The drawing under review shows one solid part. Ordinate dimensions are in mm from its lowest x, y, z. A direction names the side the tool comes from. Give positions to 0.01 mm unless a question says otherwise; leave off trailing zeros. Write each loop counter-clockwise with the first axis right and the second up, starting at its lowest first coordinate (ties: lowest second). Pieces come first, ordered by that corner, then holes. Notation, with made-up numbers: M 88,55.5 L 141,55.5 A18 ccw 141,77.5 Z; hole C -15.5,-28 d11. An arc over 180 degrees is marked long. Write each question's results on one line, items separated by ' | '. Start each with the question number.
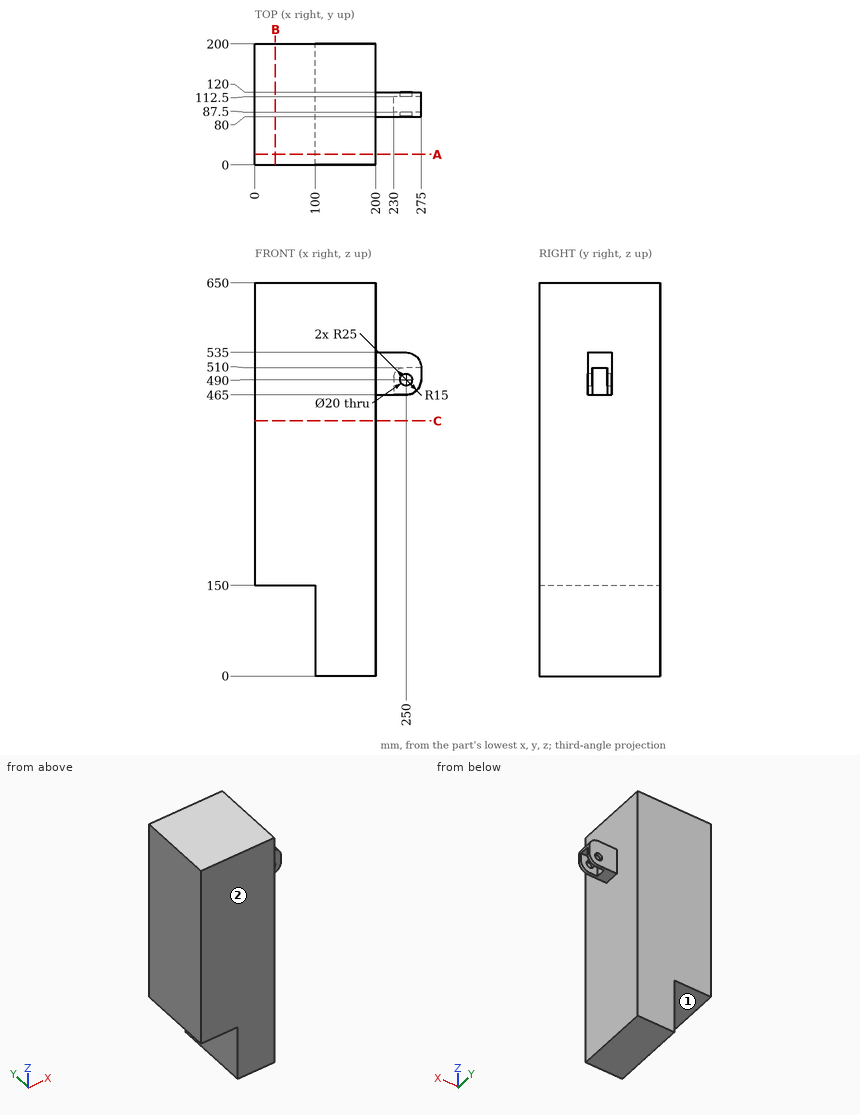
Q1. We need section C-C on z = 422. Write out the cut boundary in (x, y).
Q2. For the marked faces 1 and 2, list the 3-axis set-ups (+Z, -Z, +X, -X, +Y, -Y) from which the entire face can be reached by the end or side of a thin tool; tool diameter is ignored.
Q3. We need section A-A on y = 17.5. Write out the cut boundary in (x, z).
Q4. Wall thickness on line 1 along X through (y, z) = (82.25, 490); line 2 along X through (y, z) = (123, 406); line 3 along X through (y, z) = (178.5, 139.5): over which ranges is each line inside the solid? List them lowest first. Write a range as from..to.
Q5. For pin 1 Ø18 at (x, z) = (250, 490) entering from -Y; pin 2 Ø6 at (x, y) = (35, 150.5) entering from -Z; pin 3 Ø12 at (x, y) = (229, 109) entering from -Z; pin 4 Ø12.5 at (y, z) = (101, 476.5) entering from +X, all flat-tipped, find the tip position at first contact; note any pin that passes through.
Q6. We need section B-B on x = 34. Write out the cut boundary in (y, z), and give its area (3 significant figures).
Answer sheet:
1) outline: M 0,0 L 200,0 L 200,200 L 0,200 Z
2) face 1: -Z, -X, +Y, -Y | face 2: +Z, -Z, +X, -X, -Y
3) outline: M 0,150 L 100,150 L 100,0 L 200,0 L 200,650 L 0,650 Z
4) line 1: 0..240, 260..275 | line 2: 0..200 | line 3: 100..200
5) pin 1: through | pin 2: z = 150 | pin 3: z = 465 | pin 4: x = 230
6) outline: M 0,150 L 200,150 L 200,650 L 0,650 Z | area: 100,000 mm^2
